Could you check a few things on this model? Use its own coordinates, in mm. A direction names the side the tool comes from. Give positions to 0.01 mm unless a question says otherwise; leave off trailing zeros. Loops run counter-clockwise (first coordinate to the right, second up) from the corner with the lowest first, then second, coordinate; pieces in that order, holes last.
1. Imagine slicing it at B-B (z = 226.5). List the corners of the cut face in (x, y) for me, plus the area to 3 significant figures.
2. I need wall thicknesses on line 1 along X through (y, z) = (-24, 12); line 2 along Y through (x, z) = (6.75, 446.5); line 3 along X through (y, z) = (-6.5, 179). Which ranges of each line are inside material? Lowest first, please.
3. For P1, Ø2.5, axis at x = 0, z = 444.5, coming from the +Y side, with a flat end and sliding along its axis, tell me the tip position at first contact or that it passes through.
4. Thinking about a two-plate mould opening in X: for faces 3 (the flat face through (0, 22.81, 321)), 4 (the flat face through (0, 25.35, 321)), 5 (the flat face through (-12.7, 0, 321)), 6 (the flat face through (12.7, 0, 321)), which applies, +X half, -X half, draft (parallel to the pull), parting line (faces both ways), or undercut?
5. Imagine slicing it at A-A (y = 12). List the corners of the cut face in (x, z) for me, plus the area to 3 significant figures.
6. For faces 1 (the flat face through (10.16, 0, 321)), 2 (the flat face through (-10.4, 2, 651)), which set-ups out of +Z, -Z, +X, -X, +Y, -Y let a thin tool reach every point of the face, with its end or its side?
```python
from build123d import *

# Parameters (mm, degrees)
CROQUIS1_W              = 25.4
CROQUIS1_H              = 50.7
CROQUIS1_W_2            = 20.32
CROQUIS1_H_2            = 45.62
SALIENTE_EXTRUIR1_DEPTH = 651
CROQUIS2_R              = 2.07
CORTAR_EXTRUIR2_DEPTH   = 54


with BuildPart() as part:
    # Croquis1 → Saliente-Extruir1 (new body)
    with BuildSketch(Plane.XY):
        Rectangle(CROQUIS1_W, CROQUIS1_H)
        Rectangle(CROQUIS1_W_2, CROQUIS1_H_2, mode=Mode.SUBTRACT)
    extrude(amount=SALIENTE_EXTRUIR1_DEPTH)

    # Croquis2 → Cortar-Extruir2 (cut)
    with BuildSketch(Plane(origin=(0, 25.35, 0), x_dir=(1, 0, 0), z_dir=(0, 1, 0))):
        with Locations(Location((0, -12.7, 0), (0, 0, 270))):
            Circle(CROQUIS2_R)
        with Locations(Location((0, -38.1, 0), (0, 0, 270))):
            Circle(CROQUIS2_R)
        with Locations(Location((0, -63.5, 0), (0, 0, 270))):
            Circle(CROQUIS2_R)
        with Locations(Location((0, -88.9, 0), (0, 0, 270))):
            Circle(CROQUIS2_R)
        with Locations(Location((0, -114.3, 0), (0, 0, 270))):
            Circle(CROQUIS2_R)
        with Locations(Location((0, -139.7, 0), (0, 0, 270))):
            Circle(CROQUIS2_R)
        with Locations(Location((0, -165.1, 0), (0, 0, 270))):
            Circle(CROQUIS2_R)
        with Locations(Location((0, -190.5, 0), (0, 0, 270))):
            Circle(CROQUIS2_R)
        with Locations(Location((0, -215.9, 0), (0, 0, 270))):
            Circle(CROQUIS2_R)
        with Locations(Location((0, -241.3, 0), (0, 0, 270))):
            Circle(CROQUIS2_R)
        with Locations(Location((0, -266.7, 0), (0, 0, 270))):
            Circle(CROQUIS2_R)
        with Locations(Location((0, -292.1, 0), (0, 0, 270))):
            Circle(CROQUIS2_R)
        with Locations(Location((0, -317.5, 0), (0, 0, 270))):
            Circle(CROQUIS2_R)
        with Locations(Location((0, -342.9, 0), (0, 0, 270))):
            Circle(CROQUIS2_R)
        with Locations(Location((0, -368.3, 0), (0, 0, 270))):
            Circle(CROQUIS2_R)
        with Locations(Location((0, -393.7, 0), (0, 0, 270))):
            Circle(CROQUIS2_R)
        with Locations(Location((0, -419.1, 0), (0, 0, 270))):
            Circle(CROQUIS2_R)
        with Locations(Location((0, -444.5, 0), (0, 0, 270))):
            Circle(CROQUIS2_R)
        with Locations(Location((0, -469.9, 0), (0, 0, 270))):
            Circle(CROQUIS2_R)
        with Locations(Location((0, -495.3, 0), (0, 0, 270))):
            Circle(CROQUIS2_R)
        with Locations(Location((0, -520.7, 0), (0, 0, 270))):
            Circle(CROQUIS2_R)
        with Locations(Location((0, -546.1, 0), (0, 0, 270))):
            Circle(CROQUIS2_R)
        with Locations(Location((0, -571.5, 0), (0, 0, 270))):
            Circle(CROQUIS2_R)
        with Locations(Location((0, -596.9, 0), (0, 0, 270))):
            Circle(CROQUIS2_R)
        with Locations(Location((0, -622.3, 0), (0, 0, 270))):
            Circle(CROQUIS2_R)
        with Locations(Location((0, -647.7, 0), (0, 0, 270))):
            Circle(CROQUIS2_R)
    extrude(amount=-CORTAR_EXTRUIR2_DEPTH, mode=Mode.SUBTRACT)


solid = part.part
```
Derived:
1. outline: (-12.7, -25.35) - (12.7, -25.35) - (12.7, 25.35) - (-12.7, 25.35) - close; hole (-10.16, -22.81) - (10.16, -22.81) - (10.16, 22.81) - (-10.16, 22.81) - close
1. area: 361 mm2
2. line 1: x = -12.7 to -1.95, 1.95 to 12.7
2. line 2: y = -25.35 to -22.81, 22.81 to 25.35
2. line 3: x = -12.7 to -10.16, 10.16 to 12.7
3. P1: passes through
4. face 3: undercut
4. face 4: draft
4. face 5: -X half
4. face 6: +X half
5. outline: (-12.7, 0) - (-10.16, 0) - (-10.16, 651) - (-12.7, 651) - close; (10.16, 0) - (12.7, 0) - (12.7, 651) - (10.16, 651) - close
5. area: 3,310 mm2
6. face 1: +Z, -Z
6. face 2: +Z, +X, -X, +Y, -Y
